from build123d import *

# Parameters (mm, degrees)
SKETCH2_R           = 4
BOSS_EXTRUDE1_DEPTH = 6
SKETCH3_R           = 4.99
CUT_EXTRUDE1_DEPTH  = 3


with BuildPart() as part:
    # Sketch2 → Boss-Extrude1 (new body)
    with BuildSketch(Plane(origin=(0, 0, 0), x_dir=(0, 0, -1), z_dir=(1, 0, 0))):
        with BuildLine():
            Line((-47.806823021, 48.229255235), (-35.735718863, 42.04148953))
            ThreePointArc((-35.735718863, 42.04148953), (-30.003159714, 40.51527432), (-24.153212483, 41.5))
            Line((-24.153212483, 41.5), (-11.349364905, 41.5))
            Line((-11.349364905, 41.5), (-11.349364905, 29.5))
            Line((-11.349364905, 29.5), (-25.79380935, 22.333548668))
            ThreePointArc((-25.79380935, 22.333548668), (-29.761404347, 21.510618078), (-33.623291754, 22.737341551))
            Line((-33.623291754, 22.737341551), (-54.739685992, 36.082673857))
            ThreePointArc((-54.739685992, 36.082673857), (-57.079434827, 45.469938354), (-47.806823021, 48.229255235))
        make_face()
        with Locations((-51, 42)):
            Circle(SKETCH2_R, mode=Mode.SUBTRACT)
        with Locations((-29.349364905, 29.5)):
            Circle(SKETCH2_R, mode=Mode.SUBTRACT)
    extrude(amount=BOSS_EXTRUDE1_DEPTH)

    # Sketch3 → Cut-Extrude1 (cut)
    with BuildSketch(Plane.ZY):
        with Locations((51, 42)):
            Circle(SKETCH3_R)
    extrude(amount=-CUT_EXTRUDE1_DEPTH, mode=Mode.SUBTRACT)


solid = part.part
Input: part model. Units: mm. Frame: model coordinates. A direction names the side the tool comes from. Round coordinates to 2 decimals unless told otherwise and drop trailing zeros. Loops run counter-clockwise (first coordinate to the right, second up) from the corner with the lowest first, then second, coordinate; pieces in that order, holes last. Notation, with made-up numbers: M 72.25,36 L 130.25,36 A25 ccw 130.25,66 Z; hole C -5.5,4 d2. An arc over 180 degrees is marked long. Answer as CSV lines item,"result". Start each with the question number.
(1) Line query: line 1 (Y direction, x = 1.8, z = 51); line 2 (Z direction, x = 4.95, y = 32.25); line 3 (Z direction, x = 4.55, y = 26.5). Output: solid intervals per line, ascending. Write a range as [from, to].
(2) Reachability of faces 1 (the flat face through (3, 41.5, 18)), 2 (the cylindrical face through (2.958, 21.508, 29.704)), 3 (the flat face through (3, 44, 47)) from +Z, -Z, +X, -X, +Y, -Y: full face, straight path, thin tool, end or side. Return the list, or none.
(3) First-contact query: pin 1 (1 mm diameter, centred on x = 1, z = 46.5, fed in from -Y). Flat tip, straight axial feed; report the tip coordinate or a pass-through.
(4) Draft query along Y for faces 4 (the flat face through (3, 36, 11.349)), 5 (the cylindrical face through (4.48, 44.7, 53.95)), 6 (the flat face through (3, 45.2, 41.9)). Return one class per face: released by +Y, released by -Y, zero draft, split by the parting line, or undercut.
(5) Section B-B, the plane x = 5.4. Output: boundary loops of the cut face in (y, z).
(6) Section C-C, the plane z = 51. Output: boundary loops of the cut face in (x, y).
(7) Section D-D, the plane x = 1.5. Output: boundary loops of the cut face in (y, z).
(8) Section A-A, the plane y = 26.5. Output: boundary loops of the cut face in (x, z).
Values found:
1,line 1,"y = [33.72, 37.01], [46.99, 49]"
1,line 2,"z = [11.35, 26.44], [32.25, 48.68]"
1,line 3,"z = [17.4, 26.7], [32, 39.58]"
2,face 1,"-Z, +X, -X, +Y"
2,face 2,"+X, -X, -Y"
2,face 3,"-X"
3,pin 1,"stops at y = 30.56"
4,face 4,"zero draft"
4,face 5,"undercut"
4,face 6,"released by +Y"
5,outline,"M 22.33,25.79 L 29.5,11.35 L 41.5,11.35 L 41.5,24.15 A14 cw 42.04,35.74 L 48.23,47.81 A7 ccw 36.08,54.74 L 22.74,33.62 A8 ccw Z; hole C 29.5,29.35 d8; hole C 42,51 d8"
6,outline,"M 0,33.72 L 6,33.72 L 6,38 L 3,38 L 3,37.01 L 0,37.01 Z; M 0,46.99 L 3,46.99 L 3,46 L 6,46 L 6,49 L 0,49 Z"
7,outline,"M 22.33,25.79 L 29.5,11.35 L 41.5,11.35 L 41.5,24.15 A14 cw 42.04,35.74 L 48.23,47.81 A7 ccw 36.08,54.74 L 22.74,33.62 A8 ccw Z; hole C 29.5,29.35 d8; hole C 42,51 d9.98"
8,outline,"M 0,17.4 L 6,17.4 L 6,26.7 L 0,26.7 Z; M 0,32 L 6,32 L 6,39.58 L 0,39.58 Z"
